from build123d import *

# Parameters (mm, degrees)
F0_R     = 135.763
F0_R_2   = 5.461
F1_DEPTH = 1.0922


with BuildPart() as f1:
    # F0 (on Front) → F1 (new body)
    with BuildSketch(Plane.XZ):
        with BuildLine():
            ThreePointArc((-49.730106, 103.42222), (-50.285138, 101.441998), (-51.788522, 100.038724))
            ThreePointArc((-51.788522, 100.038724), (-112.649, 0), (-51.788522, -100.038724))
            ThreePointArc((-51.788522, -100.038724), (-50.285138, -101.441998), (-49.730106, -103.42222))
            Line((-49.730106, -103.42222), (-49.730106, -109.893576))
            ThreePointArc((-49.730106, -109.893576), (-49.096339, -111.997773), (-47.405883, -113.401933))
            ThreePointArc((-47.405883, -113.401933), (-32.475361, -118.611287), (-16.996183, -121.844388))
            ThreePointArc((-16.996183, -121.844388), (-15.00917, -121.594865), (-13.423186, -120.372107))
            Line((-13.423186, -120.372107), (-8.61764, -114.025335))
            ThreePointArc((-8.61764, -114.025335), (-7.193966, -112.873921), (-5.397561, -112.519614))
            ThreePointArc((-5.397561, -112.519614), (112.649, 0), (-5.397561, 112.519614))
            ThreePointArc((-5.397561, 112.519614), (-7.193966, 112.873921), (-8.61764, 114.025335))
            Line((-8.61764, 114.025335), (-13.423186, 120.372107))
            ThreePointArc((-13.423186, 120.372107), (-15.00917, 121.594865), (-16.996183, 121.844388))
            ThreePointArc((-16.996183, 121.844388), (-32.475361, 118.611287), (-47.405883, 113.401933))
            ThreePointArc((-47.405883, 113.401933), (-49.096339, 111.997773), (-49.730106, 109.893576))
            Line((-49.730106, 109.893576), (-49.730106, 103.42222))
        make_face()
        Circle(F0_R)
        with Locations((-73.155753, -100.690255)):
            Circle(F0_R_2, mode=Mode.SUBTRACT)
        with Locations((-118.368494, -38.460255)):
            Circle(F0_R_2, mode=Mode.SUBTRACT)
        with Locations((0, -124.46)):
            Circle(F0_R_2, mode=Mode.SUBTRACT)
        with Locations((73.155753, -100.690255)):
            Circle(F0_R_2, mode=Mode.SUBTRACT)
        with Locations((118.368494, -38.460255)):
            Circle(F0_R_2, mode=Mode.SUBTRACT)
        with Locations((-118.368494, 38.460255)):
            Circle(F0_R_2, mode=Mode.SUBTRACT)
        with Locations((-73.155753, 100.690255)):
            Circle(F0_R_2, mode=Mode.SUBTRACT)
        with BuildLine():
            ThreePointArc((-51.788522, -100.038724), (-112.649, 0), (-51.788522, 100.038724))
            ThreePointArc((-51.788522, 100.038724), (-50.285138, 101.441998), (-49.730106, 103.42222))
            Line((-49.730106, 103.42222), (-49.730106, 109.893576))
            ThreePointArc((-49.730106, 109.893576), (-49.096339, 111.997773), (-47.405883, 113.401933))
            ThreePointArc((-47.405883, 113.401933), (-32.475361, 118.611287), (-16.996183, 121.844388))
            ThreePointArc((-16.996183, 121.844388), (-15.00917, 121.594865), (-13.423186, 120.372107))
            Line((-13.423186, 120.372107), (-8.61764, 114.025335))
            ThreePointArc((-8.61764, 114.025335), (-7.193966, 112.873921), (-5.397561, 112.519614))
            ThreePointArc((-5.397561, 112.519614), (112.649, 0), (-5.397561, -112.519614))
            ThreePointArc((-5.397561, -112.519614), (-7.193966, -112.873921), (-8.61764, -114.025335))
            Line((-8.61764, -114.025335), (-13.423186, -120.372107))
            ThreePointArc((-13.423186, -120.372107), (-15.00917, -121.594865), (-16.996183, -121.844388))
            ThreePointArc((-16.996183, -121.844388), (-32.475361, -118.611287), (-47.405883, -113.401933))
            ThreePointArc((-47.405883, -113.401933), (-49.096339, -111.997773), (-49.730106, -109.893576))
            Line((-49.730106, -109.893576), (-49.730106, -103.42222))
            ThreePointArc((-49.730106, -103.42222), (-50.285138, -101.441998), (-51.788522, -100.038724))
        make_face(mode=Mode.SUBTRACT)
        with Locations((118.368494, 38.460255)):
            Circle(F0_R_2, mode=Mode.SUBTRACT)
        with Locations((0, 124.46)):
            Circle(F0_R_2, mode=Mode.SUBTRACT)
        with Locations((73.155753, 100.690255)):
            Circle(F0_R_2, mode=Mode.SUBTRACT)
    extrude(amount=F1_DEPTH)


solid = f1.part
Work out the finished part from the listing and answer in its coordinate system (mm). A direction names the side the tool comes from. Round coordinates to 2 decimals unless told otherwise and drop trailing zeros. Write each loop counter-clockwise with the first axis right and the second up, starting at its lowest first coordinate (ties: lowest second). Pieces come first, ordered by that corner, then holes. Notation, with made-up numbers: (22.25, -28) -> (62.25, -28) arc R28 ccw to (62.25, -5) -> close; hole circle Ø4 at (12, 51.25). An arc over 180 degrees is marked (long way). Write each question's results on one line, items separated by ' | '.
Item 1: Which of the six approach directions +Z, -Z, +X, -X, +Y, -Y give full straight-line access (tool end or side, diameter ignored) to faces 1 (the face through (-32.26, -0.54, -118.67)), 2 (the face through (30, -1.092, -110))?
Result set:
face 1: +Y, -Y | face 2: +Z, -Z, +X, -X, -Y
Item 2: A cutting plane is placed at C-C, the plane y = -0.7. Count the separate pieces of the cut face and the enclosed holes in it, plus the area to 3 significant figures.
Result set:
separate pieces: 1 | enclosed holes: 11 | area: 16,300 mm^2
Item 3: A cutting plane is placed at A-A, the plane z = 0. Determine the outline of the cut face in (x, y), plus the area to 3 significant figures.
Result set:
outline: (-135.76, -1.09) -> (-112.65, -1.09) -> (-112.65, 0) -> (-135.76, 0) -> close; (112.65, -1.09) -> (135.76, -1.09) -> (135.76, 0) -> (112.65, 0) -> close | area: 50.5 mm^2
Item 4: A cutting plane is placed at D-D, the plane x = -118. Determine the outline of the cut face in (y, z), plus the area to 3 significant figures.
Result set:
outline: (-1.09, -67.14) -> (0, -67.14) -> (0, -43.91) -> (-1.09, -43.91) -> close; (-1.09, -33.01) -> (0, -33.01) -> (0, 33.01) -> (-1.09, 33.01) -> close; (-1.09, 43.91) -> (0, 43.91) -> (0, 67.14) -> (-1.09, 67.14) -> close | area: 123 mm^2
Item 5: Find the intervals of material crossed by line 1 along X through (y, z) = (-0.3, 35.5); line 2 along Z through (x, y) = (121.5, -0.4); line 3 along X through (y, z) = (-0.35, -39.5), in increasing order. Write a range as [from, to].
Result set:
line 1: [-131.04, -122.96], [-113.78, -106.91], [106.91, 113.78], [122.96, 131.04] | line 2: [-60.58, -42.93], [-33.99, 33.99], [42.93, 60.58] | line 3: [-129.89, -123.73], [-113.01, -105.5], [105.5, 113.01], [123.73, 129.89]
Item 6: A cutting plane is placed at B-B, the plane x = 94. Determine the outline of the cut face in (y, z).
Result set:
outline: (-1.09, -97.96) -> (0, -97.96) -> (0, -62.08) -> (-1.09, -62.08) -> close; (-1.09, 62.08) -> (0, 62.08) -> (0, 97.96) -> (-1.09, 97.96) -> close
Item 7: A flat-ended cylindrical pin translates along its axis: P1, Ø0.5, axis at y = -0.5, z = -107.5, coming from the +X side. Find the tip coordinate at first contact, or state that the pin passes through.
Result set:
P1: x = 83.24
Item 8: The mould has two halves that part along Z. Classify faces 3 (the face through (-1.18, -0.54, -129.79)), 4 (the face through (-107.737, -0.538, -82.61)), 5 (the face through (30, 0, -110)): +Z half, -Z half, draft (parallel to the pull), parting line (faces both ways), or undercut.
Result set:
face 3: undercut | face 4: parting line | face 5: draft
